Could you check a few things on this model? Use its own coordinates, in mm. A direction names the side the tool comes from. Coordinates: 2 decimals unless noted, no trailing zeros. Write each loop counter-clockwise with the first axis right and the second up, starting at its lowest first coordinate (ties: lowest second). Pieces come first, ordered by that corner, then holes.
Item 1: I want a section at B-B on x = -20.5. Please give me the cut outline in (y, z).
Item 2: For P1, Ø4.5, axis at x = -7.5, y = -18.19, coming from the +Z side; P2, Ø4, axis at y = -3.5, z = 11, coming from the -X side; P3, Ø4, axis at x = -8.5, z = 4.5, coming from the -Y side; P4, Ø1.5, axis at x = 5.5, y = -3.5, coming from the -Z side, each with a flat end and sliding along its axis, tell me the tip position at first contact or that it passes through.
Item 3: Thinking about a two-plate mould opening in X: for faces 1 (the flat face through (22.415, 8.537, 11.545)), 2 (the flat face through (-20, -1.738, 5)), 3 (the flat face through (-32, 7, 7)), 4 (the flat face through (-22.585, 8.537, 11.545)), which applies, +X half, -X half, draft (parallel to the pull), parting line (faces both ways), or undercut?
Item 4: I want a section at A-A on x = -7.5. Please give me the cut outline in (y, z).
Item 5: If I drill on probe 1 along Y at (x, z) = (7.5, 0.85); probe 2 along X at (y, z) = (9, 11.75); probe 3 along X at (y, z) = (5, 12.5), over which ranges is the centre line in solid material (lowest first)?
Item 6: Which directions (+Z, -Z, +X, -X, +Y, -Y) give clear straight access to the entire face, cutting with the end or side of a thin tool? Please do faces 5 (the flat face through (2, -6, 13)), 6 (the flat face through (1.755, -1.558, 6.204)), 7 (the cylindrical face through (-6.136, 8.063, 0.912)), 8 (the flat face through (5.45, -6, 11)).
Item 7: I want a section at C-C on z = 4.5. State how many separate pieces and enclosed holes the cut face has, then the cut area to 3 significant figures.
from build123d import *

# Parameters (mm, degrees)
F0_W            = 28.0605573207
F0_H            = 17.1019586477
F1_DEPTH        = 3
F3_DEPTH        = 32
F3_DEPTH_BACK   = 32
F4_DEPTH        = 25
F5_W            = 28.0605573207
F5_H            = 17.0454510609
F5_H_2          = 8.3564384666
F6_REACH        = 49.2047839512
F5_R            = 6.05
F7_DEPTH        = 3
F9_DEPTH        = 10
F10_D           = 3.7
F10_CSINK_D     = 6
F10_CSINK_ANGLE = 90
F12_DEPTH       = 25
F13_DEPTH       = 25
F14_DEPTH       = 5


# Not quite as in the source:
# - a feature names something its author has since deleted; it is built from what else it names


with BuildPart() as f1:
    # F0 (on Top) → F1 (new body)
    with BuildSketch(Plane.XY):
        with BuildLine():
            Line((-19.0302786604, -1.7378998397), (-14.0302786604, -1.7378998397))
            Line((-14.0302786604, -1.7378998397), (-14.0302786604, 15.3640588081))
            Line((-14.0302786604, 15.3640588081), (-27, 15.3640588081))
            ThreePointArc((-27, 15.3640588081), (-30.5355339059, 13.899592714), (-32, 10.3640588081))
            Line((-32, 10.3640588081), (-32, 3.2621001603))
            ThreePointArc((-32, 3.2621001603), (-30.5355339059, -0.2734337456), (-27, -1.7378998397))
            Line((-27, -1.7378998397), (-20.8602603525, -1.7378998397))
            Line((-20.8602603525, -1.7378998397), (-19.0302786604, -1.7378998397))
        make_face()
        with BuildLine():
            ThreePointArc((-14.0302786604, -20.1735929717), (-12.5658125663, -23.7091268776), (-9.0302786604, -25.1735929717))
            Line((-9.0302786604, -25.1735929717), (9.0302786604, -25.1735929717))
            ThreePointArc((9.0302786604, -25.1735929717), (12.5658125663, -23.7091268776), (14.0302786604, -20.1735929717))
            Line((14.0302786604, -20.1735929717), (14.0302786604, -6.7378998397))
            Line((14.0302786604, -6.7378998397), (14.0302786604, -1.7378998397))
            Line((14.0302786604, -1.7378998397), (-14.0302786604, -1.7378998397))
            Line((-14.0302786604, -1.7378998397), (-14.0302786604, -6.7378998397))
            Line((-14.0302786604, -6.7378998397), (-14.0302786604, -20.1735929717))
        make_face()
        with BuildLine():
            Line((14.0302786604, 15.3640588081), (14.0302786604, -1.7378998397))
            Line((14.0302786604, -1.7378998397), (19.0302786604, -1.7378998397))
            Line((19.0302786604, -1.7378998397), (21.6872710735, -1.7378998397))
            Line((21.6872710735, -1.7378998397), (27, -1.7378998397))
            ThreePointArc((27, -1.7378998397), (30.5355339059, -0.2734337456), (32, 3.2621001603))
            Line((32, 3.2621001603), (32, 10.3640588081))
            ThreePointArc((32, 10.3640588081), (30.5355339059, 13.899592714), (27, 15.3640588081))
            Line((27, 15.3640588081), (14.0302786604, 15.3640588081))
        make_face()
        with Locations((0, 6.8130794842)):
            Rectangle(F0_W, F0_H)
        with BuildLine():
            ThreePointArc((-19.0302786604, -1.7378998397), (-15.4947447544, -3.2023659338), (-14.0302786604, -6.7378998397))
            Line((-14.0302786604, -6.7378998397), (-14.0302786604, -1.7378998397))
            Line((-14.0302786604, -1.7378998397), (-19.0302786604, -1.7378998397))
        make_face()
        with BuildLine():
            Line((14.0302786604, -1.7378998397), (14.0302786604, -6.7378998397))
            ThreePointArc((14.0302786604, -6.7378998397), (15.4947447544, -3.2023659338), (19.0302786604, -1.7378998397))
            Line((19.0302786604, -1.7378998397), (14.0302786604, -1.7378998397))
        make_face()
    extrude(amount=F1_DEPTH)

    # F2 (on Right) → F3 (join, two sides)
    with BuildSketch(Plane.YZ) as f3_sk:
        with BuildLine():
            Line((-1.7378998397, 8), (-1.7378998397, 3))
            Line((-1.7378998397, 3), (15.3640588081, 3))
            Line((15.3640588081, 3), (15.3640588081, 16.1534193361))
            ThreePointArc((15.3640588081, 16.1534193361), (14.2866836868, 17.9278948454), (12.2152954749, 17.7905945877))
            Line((12.2152954749, 17.7905945877), (-1.7378998397, 8))
        make_face()
    extrude(amount=F3_DEPTH)
    extrude(f3_sk.sketch, amount=-F3_DEPTH_BACK)

    # F4 (cut): faces of the model
    f4_faces = [f1.faces().sort_by_distance(p)[0] for p in [
        (-30.8831603053, 14.2472191133, 3),
        (-30.8831603053, -0.621060145, 3),
        (30.8831603053, -0.621060145, 3),
        (30.8831603053, 14.2472191133, 3),
    ]]
    extrude(f4_faces, amount=-F4_DEPTH, mode=Mode.SUBTRACT)

    f6_end = Plane(origin=(0, -13.1098018859, 3), x_dir=(1, 0, 0), z_dir=(0, 0, 1))
    # F5 (on face) → F6 (cut, up to a plane its end follows)
    with BuildSketch(Plane(origin=(0, -4.334811805, 6.177814353), x_dir=(1, 0, 0), z_dir=(0, -0.5743816666, 0.8185876258))):
        with Locations((0, 11.6951555593)):
            Rectangle(F5_W, F5_H)
        Polygon((14.0302786604, -5.0207045861), (14.0302786604, 0), (14.0302786604, 3.1724300289), (-14.0302786604, 3.1724300289), (-14.0302786604, 0), (-14.0302786604, -5.0207045861), align=None)
        with Locations((0, 24.396100323)):
            Rectangle(F5_W, F5_H_2)
    f6_long = extrude(amount=-F6_REACH, mode=Mode.PRIVATE)
    add(split(f6_long, bisect_by=f6_end, keep=Keep.TOP, mode=Mode.PRIVATE), mode=Mode.SUBTRACT)

    # F5 (on face) → F7 (cut)
    with BuildSketch(Plane(origin=(0, -4.334811805, 6.177814353), x_dir=(1, 0, 0), z_dir=(0, -0.5743816666, 0.8185876258))):
        with Locations((22.5, 13.5350767523)):
            Circle(F5_R)
        with Locations((-22.5, 13.5350767523)):
            Circle(F5_R)
    extrude(amount=-F7_DEPTH, mode=Mode.SUBTRACT)

    # F8 (on face) → F9 (join)
    with BuildSketch(Plane.XY.offset(3)):
        with BuildLine():
            add(Edge.make_bspline(
                [(3.439653721, 14.4599989291), (4.0052184257, 14.1775319538), (4.2384614527, 13.0214622017), (5.1246291924, 10.2048677906), (5.4504108833, 9.003783584)],
                knots=[0, 0, 0, 0, 0.1106519752, 0.1831613583, 0.1831613583, 0.1831613583, 0.1831613583], degree=3))
            add(Edge.make_bspline(
                [(-2.425625543, 2.1165073176), (-2.6128697036, 2.4416064205), (-3.7900282508, 5.4402549428), (-0.4138105091, 14.2334908767), (2.8259898176, 14.7664886821), (3.439653721, 14.4599989291)],
                knots=[0.6187512381, 0.6187512381, 0.6187512381, 0.6187512381, 0.6507091383, 0.8799374811, 1, 1, 1, 1], degree=3))
            add(Edge.make_bspline(
                [(6.2951599905, 3.2293955823), (6.2536285053, 2.7551424943), (5.7362561971, 0.3058795284), (1.5238317893, -0.5897867433), (-1.6783380052, 0.8190435823), (-2.425625543, 2.1165073176)],
                knots=[0.3006282955, 0.3006282955, 0.3006282955, 0.3006282955, 0.3342495888, 0.491207925, 0.6187512381, 0.6187512381, 0.6187512381, 0.6187512381], degree=3))
            Line((6.2951599905, 3.2293955823), (6.3205224566, 4.054668216))
            ThreePointArc((6.3205224566, 4.054668216), (4.5453166658, 6.2936120697), (5.4504108833, 9.003783584))
        make_face()
        with BuildLine():
            add(Edge.make_bspline(
                [(6.2951599905, 3.2293955823), (6.2536285053, 2.7551424943), (5.7362561971, 0.3058795284), (1.5238317893, -0.5897867433), (-1.6783380052, 0.8190435823), (-2.425625543, 2.1165073176)],
                knots=[0.3006282955, 0.3006282955, 0.3006282955, 0.3006282955, 0.3342495888, 0.491207925, 0.6187512381, 0.6187512381, 0.6187512381, 0.6187512381], degree=3))
            Line((-2.425625543, 2.1165073176), (-2.4419164115, 1.5864165937))
            ThreePointArc((-2.4419164115, 1.5864165937), (-1.6394334925, -0.5495415445), (0.4334442969, -1.5032048363))
            Line((0.4334442969, -1.5032048363), (3.1138092408, -1.6133925553))
            ThreePointArc((3.1138092408, -1.6133925553), (5.2808377949, -0.8120256781), (6.2356171285, 1.2919225271))
            Line((6.2356171285, 1.2919225271), (6.2951599905, 3.2293955823))
        make_face()
        with BuildLine():
            add(Edge.make_bspline(
                [(6.3205224566, 4.054668216), (6.3259320308, 3.7685769845), (6.3182004896, 3.4924978464), (6.2951599905, 3.2293955823)],
                knots=[0.2819761483, 0.2819761483, 0.2819761483, 0.2819761483, 0.3006282955, 0.3006282955, 0.3006282955, 0.3006282955], degree=3))
            Line((6.3205224566, 4.054668216), (6.2951599905, 3.2293955823))
        make_face()
        with BuildLine():
            Line((5.7109985458, -15.7787108495), (5.7995937264, -12.895900563))
            add(Edge.make_bspline(
                [(5.7995937264, -12.895900563), (5.6014543432, -11.957203972), (5.2341196587, -10.747475142), (4.4402012509, -10.0397747357), (4.2548362634, -9.909795659)],
                knots=[0.078280994, 0.078280994, 0.078280994, 0.078280994, 0.1532878364, 0.173703161, 0.173703161, 0.173703161, 0.173703161], degree=3))
            ThreePointArc((4.2548362634, -9.909795659), (3.5782527554, -9.6387470487), (2.8562729835, -9.5388581041))
            Line((2.8562729835, -9.5388581041), (0.2851764489, -9.4984770116))
            add(Edge.make_bspline(
                [(0.2851764489, -9.4984770116), (0.1886962517, -9.5257281074), (-1.4223255568, -10.024145371), (-2.5699293228, -11.1174611467), (-2.8875198131, -12.9131313678)],
                knots=[0.2910251466, 0.2910251466, 0.2910251466, 0.2910251466, 0.2995550952, 0.4354391583, 0.4354391583, 0.4354391583, 0.4354391583], degree=3))
            Line((-2.8875198131, -12.9131313678), (-2.9514315077, -14.9927624413))
            add(Edge.make_bspline(
                [(-2.9514315077, -14.9927624413), (-2.7153775465, -18.0022293403), (-0.7781826645, -23.3457780002), (1.0082290092, -25.0100423947), (1.4971567675, -25.1735929717)],
                knots=[0.4816763185, 0.4816763185, 0.4816763185, 0.4816763185, 0.6642562574, 0.7348765677, 0.7348765677, 0.7348765677, 0.7348765677], degree=3))
            Line((1.4971567675, -25.1735929717), (2.2805444633, -25.1735929717))
            add(Edge.make_bspline(
                [(2.2805444633, -25.1735929717), (3.0961818535, -24.8930551973), (4.5940584593, -22.6765141), (5.2897590721, -21.2040650633), (5.4504108833, -20.3776246156)],
                knots=[0.7729673791, 0.7729673791, 0.7729673791, 0.7729673791, 0.8930756087, 1, 1, 1, 1], degree=3))
            ThreePointArc((5.4504108833, -20.3776246156), (4.5048044555, -18.0172041338), (5.7109985458, -15.7787108495))
        make_face()
        with BuildLine():
            add(Edge.make_bspline(
                [(5.7995937264, -12.895900563), (5.6014543432, -11.957203972), (5.2341196587, -10.747475142), (4.4402012509, -10.0397747357), (4.2548362634, -9.909795659)],
                knots=[0.078280994, 0.078280994, 0.078280994, 0.078280994, 0.1532878364, 0.173703161, 0.173703161, 0.173703161, 0.173703161], degree=3))
            Line((5.7995937264, -12.895900563), (5.8077457332, -12.6306413387))
            ThreePointArc((5.8077457332, -12.6306413387), (5.414657568, -11.0514138893), (4.2548362634, -9.909795659))
        make_face()
        with BuildLine():
            add(Edge.make_bspline(
                [(0.2851764489, -9.4984770116), (0.1886962517, -9.5257281074), (-1.4223255568, -10.024145371), (-2.5699293228, -11.1174611467), (-2.8875198131, -12.9131313678)],
                knots=[0.2910251466, 0.2910251466, 0.2910251466, 0.2910251466, 0.2995550952, 0.4354391583, 0.4354391583, 0.4354391583, 0.4354391583], degree=3))
            Line((0.2851764489, -9.4984770116), (0.173816477, -9.4967280157))
            ThreePointArc((0.173816477, -9.4967280157), (-1.9448049821, -10.32637036), (-2.8718793694, -12.4042049027))
            Line((-2.8718793694, -12.4042049027), (-2.8875198131, -12.9131313678))
        make_face()
        with BuildLine():
            add(Edge.make_bspline(
                [(1.4971567675, -25.1735929717), (1.7608720486, -25.2618080212), (2.0218753444, -25.2625619913), (2.2805444633, -25.1735929717)],
                knots=[0.7348765677, 0.7348765677, 0.7348765677, 0.7348765677, 0.7729673791, 0.7729673791, 0.7729673791, 0.7729673791], degree=3))
            Line((2.2805444633, -25.1735929717), (1.4971567675, -25.1735929717))
        make_face()
    extrude(amount=F9_DEPTH)

    # F10 (through all)
    with Locations(Plane.XY.offset(3)):
        with Locations((-7.5, 6.8130794842), (-7.5, -18.1869205158), (7.5, 6.8130794842), (7.5, -18.1869205158)):
            CounterSinkHole(F10_D / 2, F10_CSINK_D / 2, counter_sink_angle=F10_CSINK_ANGLE)

    # F11 (on Front) → F12 (join)
    with BuildSketch(Plane.XZ):
        with BuildLine():
            Line((-2.9514315077, 9.5), (5.4504108833, 9.5))
            Line((5.4504108833, 9.5), (5.4504108833, 13))
            add(Edge.make_bspline(
                [(5.4504108833, 13), (2.649796753, 13), (-0.1508173774, 13), (-2.9514315077, 13)],
                knots=[0.0010524799, 0.0010524799, 0.0010524799, 0.0010524799, 0.9996431059, 0.9996431059, 0.9996431059, 0.9996431059], degree=3))
            Line((-2.9514315077, 13), (-2.9514315077, 9.5))
        make_face()
    extrude(amount=F12_DEPTH)

    # F13 (cut): faces of the model
    f13_faces = [f1.faces().sort_by_distance(p)[0] for p in [
        (-1.8145257216, -22.2530122303, 9.5),
        (4.6195780711, -23.6613899314, 9.5),
        (5.0645605364, -18.1869205158, 9.5),
        (4.6195780711, -23.6613899314, 9.5),
    ]]
    extrude(f13_faces, amount=-F13_DEPTH, mode=Mode.SUBTRACT)

    # F14 (add): a face of the model
    f14_faces = [f1.faces().sort_by_distance(p)[0] for p in [
        (-2.4980717075, 0, 11.25),
    ]]
    extrude(f14_faces, amount=F14_DEPTH)


solid = f1.part
Response values:
1. outline: (-1.74, 0) - (15.36, 0) - (15.36, 16.15) arc R2 ccw to (12.22, 17.79) - (11.42, 17.23) - (13.14, 14.78) - (3.79, 8.22) - (2.07, 10.67) - (-1.74, 8) - close
2. P1: stops at z = 2.25
2. P2: stops at x = -2.95
2. P3: stops at y = -25.17
2. P4: stops at z = 0
3. face 1: undercut
3. face 2: draft
3. face 3: -X half
3. face 4: undercut
4. outline: (-25.17, 0) - (-20.04, 0) - (-20.04, 1.85) - (-21.19, 3) - (-25.17, 3) - close; (-16.34, 0) - (4.96, 0) - (4.96, 1.85) - (3.81, 3) - (-15.19, 3) - (-16.34, 1.85) - close; (8.66, 0) - (15.36, 0) - (15.36, 3) - (9.81, 3) - (8.66, 1.85) - close
5. probe 1: y = -25.17 to -20.04, -16.34 to 4.96, 8.66 to 15.36
5. probe 2: x = -32 to -14.03, -2.04 to 5.45, 14.03 to 32
5. probe 3: x = -32 to -28.11, -16.89 to -14.03, -2.96 to 5.11, 14.03 to 16.89, 28.11 to 32
6. face 5: +Z, +Y, -Y
6. face 6: none
6. face 7: +Z, -Z
6. face 8: +Z, +X
7. separate pieces: 4
7. enclosed holes: 0
7. area: 811 mm2
